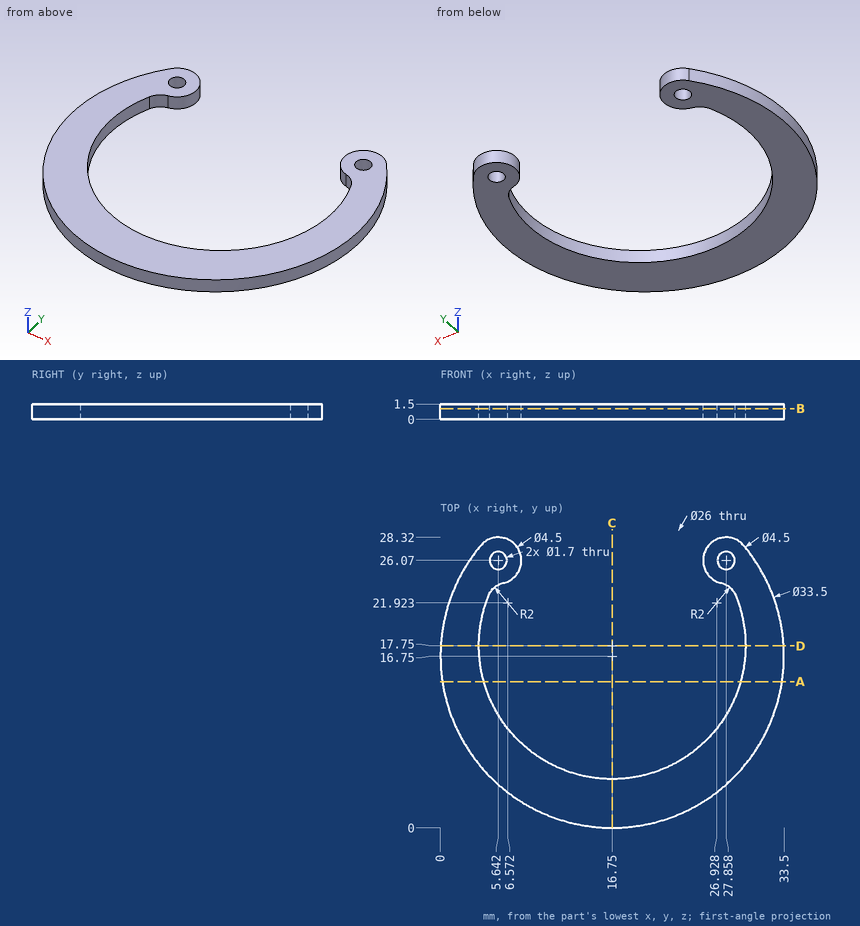
The drawing under review shows one solid part. Ordinate dimensions are in mm from its lowest x, y, z. Give positions to 0.01 mm unless a question says otherwise; leave off trailing zeros. Order: outer loops, then holes, each group sorted by start corner. A loop starts at its lowest first (then second) coordinate and runs counter-clockwise, first axis right, second up. Notation, with made-up numbers: (46, -2) -> (93, -2) arc R33 cw to (93, 28) -> close; hole circle Ø4 at (68, 73.5). An arc over 180 degrees is marked (long way). Write item = value, one per line.
1) To check wall thickness, follow L1, parallel to X at y = 7.5, z = 0.7 (1 decimal); L2, parallel to Y at x = 26, z = 1.45 (1 decimal); L3, parallel to X at y = 17.75, z = 0.4. State the ranges of each line that lie inside material, in increasing order. Write a range as from..to.
Findings:
L1 = 2.8..8.8, 24.7..30.7
L2 = 2.8..8.6, 24.8..27.3
L3 = 0.03..3.75, 29.75..33.47
2) Insertion check: pin 1 (6 mm diameter, centred on x = 22.5, y = 21, fed in from -Z). The pin has a flat end and moves straight along its axis. Give the tip position at first contact, or say it passes through.
Findings:
pin_1 = through
3) We need section C-C, the plane x = 16.75. Give the boundary of the cut face in (y, z).
Findings:
outline = (0, 0) -> (4.75, 0) -> (4.75, 1.5) -> (0, 1.5) -> close
4) We need section B-B, the plane z = 1.05. Count the separate pieces of the cut face and the enclosed holes in it, and give its area (3 significant figures).
Findings:
separate_pieces = 1
enclosed_holes = 2
area = 289 mm^2
5) We need section D-D, the plane y = 17.75. Give the boundary of the cut face in (x, z).
Findings:
outline = (0.03, 0) -> (3.75, 0) -> (3.75, 1.5) -> (0.03, 1.5) -> close; (29.75, 0) -> (33.47, 0) -> (33.47, 1.5) -> (29.75, 1.5) -> close
6) We need section A-A, the plane y = 14.25. Give the boundary of the cut face in (x, z), and give its area (3 significant figures).
Findings:
outline = (0.19, 0) -> (4.23, 0) -> (4.23, 1.5) -> (0.19, 1.5) -> close; (29.27, 0) -> (33.31, 0) -> (33.31, 1.5) -> (29.27, 1.5) -> close
area = 12.1 mm^2
